from build123d import *

# Parameters (mm, degrees)
SKETCH1_R           = 1
BOSS_EXTRUDE1_DEPTH = 5
SKETCH2_R           = 0.75
CUT_EXTRUDE1_DEPTH  = 5
CHAMFER1_SIZE2      = 2
CHAMFER1_SIZE       = 1.943358552


with BuildPart() as part:
    # Sketch1 → Boss-Extrude1 (new body)
    with BuildSketch(Plane.XY):
        with BuildLine():
            Line((63.978592029, 21.214561498), (63.978592029, 25.05586024))
            Line((63.978592029, 25.05586024), (72.058256518, 24.816727889))
            ThreePointArc((72.058256518, 24.816727889), (75.595399687, 23.198311963), (76.902246949, 19.534597706))
            Line((76.902246949, 19.534597706), (76.555916572, 13.453920838))
            ThreePointArc((76.555916572, 13.453920838), (75.36962468, 11.661641728), (76.3447433, 9.746257553))
            Line((76.3447433, 9.746257553), (76.063685342, 4.811597648))
            ThreePointArc((76.063685342, 4.811597648), (75.584983034, 3.649375801), (75.928626908, 2.440316493))
            Line((75.928626908, 2.440316493), (75.640205821, -2.623621136))
            ThreePointArc((75.640205821, -2.623621136), (74.017880394, -6.033338403), (70.473798594, -7.336256597))
            Line((70.473798594, -7.336256597), (58.930433709, -6.933153413))
            Line((58.930433709, -6.933153413), (58.930433709, -2.832883595))
            Line((58.930433709, -2.832883595), (71.435141734, -3.122466307))
            Line((71.435141734, -3.122466307), (72.093475791, 21.214561498))
            Line((72.093475791, 21.214561498), (63.978592029, 21.214561498))
        make_face()
        with Locations((73.176178498, -4.091448782)):
            Circle(SKETCH1_R, mode=Mode.SUBTRACT)
        with Locations((73.756130882, 9.746257553)):
            Circle(SKETCH1_R, mode=Mode.SUBTRACT)
    extrude(amount=BOSS_EXTRUDE1_DEPTH)

    # Sketch2 → Cut-Extrude1 (cut)
    with BuildSketch(Plane.XY.offset(5)):
        with Locations((65.076045823, -4.950719542)):
            Circle(SKETCH2_R)
        with Locations((66.046251832, 22.832345449)):
            Circle(SKETCH2_R)
    extrude(amount=-CUT_EXTRUDE1_DEPTH, mode=Mode.SUBTRACT)

    # Chamfer1
    chamfer1_edges = [part.edges().sort_by_distance(p)[0] for p in [
        (63.978592029, 25.05586024, 2.5),
    ]]
    chamfer(chamfer1_edges, length=CHAMFER1_SIZE, length2=CHAMFER1_SIZE2)


solid = part.part
Geometry check sheet. Reference: the model listing, model coordinates, mm. A direction names the side the tool comes from. Coordinates: 2 decimals unless noted, no trailing zeros. Loops run counter-clockwise (first coordinate to the right, second up) from the corner with the lowest first, then second, coordinate; pieces in that order, holes last. Notation, with made-up numbers: (87, 84.5) - (113, 84.5) arc R38 ccw to (113, 123.5) - close; hole circle Ø5 at (-26.5, 3). An arc over 180 degrees is marked (long way). Use one line per item in the form item = value. Start each with the question number.
Item 1: Gauge pin test, flat ends, axial feed: pin 1 (10 mm diameter, centred on x = 65.5, y = 7, fed in from +Z); pin 2 (1 mm diameter, centred on y = 2.5, z = 3.5, fed in from -X); pin 3 (1 mm diameter, centred on x = 70.5, z = 1, fed in from -Y); pin 4 (2 mm diameter, centred on y = 19.5, z = 1, fed in from -X). Record the tip position at first contact, or that the pin passes through.
Item 2: Thickness scan on probe 1 along Y at (x, z) = (65.5, 1); probe 2 along Y at (x, z) = (65.25, 2.55); probe 3 along Y at (x, z) = (66.5, 4.3). Record the ranges inside material, lowest first.
Item 3: Mould release check, pull along X, two halves, no side actions. Record for faces 1 (the face through (74.1, -4.47, 2.46)), 2 (the face through (75.586, 3.667, 2.465)), 3 (the face through (72, 9, 5)), 4 (the face through (58.93, -5, 2)): +X half, -X half, draft (parallel to the pull), parting line (faces both ways), or undercut.
Item 4: Section check B-B, the plane y = 17.5. Enter the section's corners in (x, z).
Item 5: Tool access check on faces 5 (the face through (68, 21.215, 2)), 6 (the face through (64.992, 24.068, 2.465)). Record the directions out of +Z, -Z, +X, -X, +Y, -Y that give a thin tool (end or side, any length) a straight path to the whole face; none if there is none.
Item 6: Section check A-A, the plane z = 1.3. Enter the section's corners in (x, y).
Item 7: Section check C-C, the plane x = 60. Enter the section's corners in (y, z), and give its area (3 significant figures).
Computed:
q1.pin_1 = through
q1.pin_2 = 71.57
q1.pin_3 = -7.34
q1.pin_4 = 72.02
q2.probe_1 = -7.16 to -5.57, -4.33 to -2.99, 21.21 to 22.32, 23.35 to 24.55
q2.probe_2 = -7.15 to -5.68, -4.22 to -2.98, 21.21 to 24.31
q2.probe_3 = -7.2 to -3.01, 21.21 to 22.24, 23.43 to 24.98
q3.face_1 = undercut
q3.face_2 = +X half
q3.face_3 = draft
q3.face_4 = -X half
q4.outline = (71.99, 0) - (76.79, 0) - (76.79, 5) - (71.99, 5) - close
q5.face_5 = +Z, -Z, -X
q5.face_6 = +Z, -Z, -X, +Y
q6.outline = (58.93, -6.93) - (70.47, -7.34) arc R5 ccw to (75.64, -2.62) - (75.93, 2.44) arc R1.92 cw to (76.06, 4.81) - (76.34, 9.75) arc R2.13 cw to (76.56, 13.45) - (76.9, 19.53) arc R5 ccw to (72.06, 24.82) - (65.98, 25) - (63.98, 23.11) - (63.98, 21.21) - (72.09, 21.21) - (71.44, -3.12) - (58.93, -2.83) - close; hole circle Ø1.5 at (65.08, -4.95); hole circle Ø1.5 at (66.05, 22.83); hole circle Ø2 at (73.18, -4.09); hole circle Ø2 at (73.76, 9.75)
q7.outline = (-6.97, 0) - (-2.86, 0) - (-2.86, 5) - (-6.97, 5) - close
q7.area = 20.6 mm2
